Geometry check sheet. Reference: the model listing, model coordinates, mm. Give positions to 0.01 mm unless a question says otherwise; leave off trailing zeros. Write each loop counter-clockwise with the first axis right and the second up, starting at its lowest first coordinate (ties: lowest second). Pieces come first, ordered by that corner, then holes. Notation, with made-up numbers: M 33,69 L 50,69 A26 cw 50,89 Z; hole C -10,23.25 d5. An arc over 180 degrees is marked long. One line per item, written item: value. Start each with the question number.
1. Scan lines: line 1 (Y direction, x = -3, z = 3.5); line 2 (Y direction, x = -4, z = 3.3). Record each from-to range of solid material in increasing order.
2. Cross-section at A-A on z = 2.8. Count the separate pieces of the cut face and the enclosed holes in it, then the cut area to 3 significant figures.
3. Cross-section at D-D on x = -3.5. Record the cut outline in (y, z).
4. Cross-section at B-B on x = 13. Record the cut outline in (y, z).
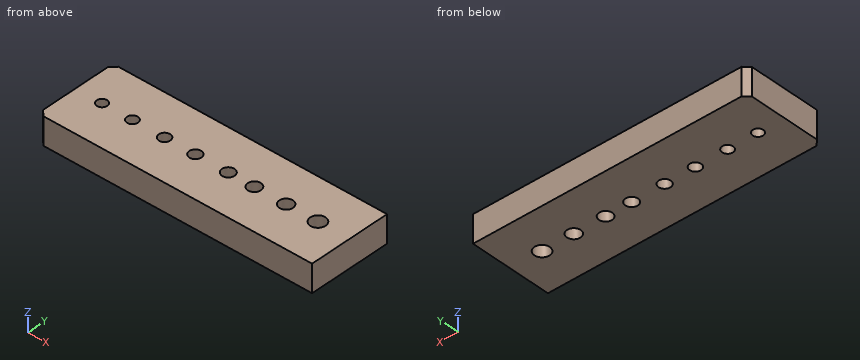
from build123d import *

# Parameters (mm, degrees)
SKETCH1_W           = 50
SKETCH1_H           = 15
BOSS_EXTRUDE1_DEPTH = 5
SKETCH2_R           = 0.95
SKETCH2_R_2         = 1
SKETCH2_R_3         = 1.05
SKETCH2_R_4         = 1.1
SKETCH2_R_5         = 1.15
SKETCH2_R_6         = 1.2
SKETCH2_R_7         = 1.25
SKETCH2_R_8         = 1.4
CUT_EXTRUDE1_DEPTH  = 6
CHAMFER1_SIZE       = 1


with BuildPart() as part:
    # Sketch1 → Boss-Extrude1 (new body)
    with BuildSketch(Plane.XY):
        Rectangle(SKETCH1_W, SKETCH1_H)
    extrude(amount=BOSS_EXTRUDE1_DEPTH)

    # Sketch2 → Cut-Extrude1 (cut, through all)
    with BuildSketch(Plane.XY.offset(5)):
        with Locations((-20.156657813, 0)):
            Circle(SKETCH2_R)
        with Locations((-14.61091069, 0)):
            Circle(SKETCH2_R_2)
        with Locations((-8.745216617, 0)):
            Circle(SKETCH2_R_3)
        with Locations((-3.128370172, 0)):
            Circle(SKETCH2_R_4)
        with Locations((2.879522545, 0)):
            Circle(SKETCH2_R_5)
        with Locations((7.643177125, 0)):
            Circle(SKETCH2_R_6)
        with Locations((13.437771876, 0)):
            Circle(SKETCH2_R_7)
        with Locations((19.232366626, 0)):
            Circle(SKETCH2_R_8)
    extrude(amount=-CUT_EXTRUDE1_DEPTH, mode=Mode.SUBTRACT)

    # Chamfer1
    chamfer1_edges = [part.edges().sort_by_distance(p)[0] for p in [
        (-25, -7.5, 2.5),
        (-25, 7.5, 2.5),
    ]]
    chamfer(chamfer1_edges, length=CHAMFER1_SIZE)


solid = part.part
Report:
1. line 1: y = -7.5 to -1.09, 1.09 to 7.5
1. line 2: y = -7.5 to -0.67, 0.67 to 7.5
2. separate pieces: 1
2. enclosed holes: 8
2. area: 716 mm^2
3. outline: M -7.5,0 L -1.04,0 L -1.04,5 L -7.5,5 Z; M 1.04,0 L 7.5,0 L 7.5,5 L 1.04,5 Z
4. outline: M -7.5,0 L -1.17,0 L -1.17,5 L -7.5,5 Z; M 1.17,0 L 7.5,0 L 7.5,5 L 1.17,5 Z
